```python
from build123d import *

# Parameters (mm, degrees)
SKETCH1_W           = 90
SKETCH1_H           = 60
BOSS_EXTRUDE1_DEPTH = 20
CUT_EXTRUDE1_DEPTH  = 61
SKETCH3_R           = 4.3
CUT_EXTRUDE2_DEPTH  = 21
SKETCH4_R           = 8.8
CUT_EXTRUDE3_DEPTH  = 10
CHAMFER1_SIZE       = 1


with BuildPart() as part:
    # Sketch1 → Boss-Extrude1 (new body)
    with BuildSketch(Plane(origin=(0, 0, 0), x_dir=(1, 0, 0), z_dir=(0, 1, 0))):
        Rectangle(SKETCH1_W, SKETCH1_H)
    extrude(amount=BOSS_EXTRUDE1_DEPTH)

    # Sketch2 → Cut-Extrude1 (cut, through all)
    with BuildSketch(Plane.XY.offset(30)):
        Polygon((28, 25), (-28, 25), (-28, 15), (-7.8, 15), (-7.8, 20), (7.8, 20), (7.8, 15), (28, 15), align=None)
    extrude(amount=-CUT_EXTRUDE1_DEPTH, mode=Mode.SUBTRACT)

    # Sketch3 → Cut-Extrude2 (cut, through all)
    with BuildSketch(Plane.XZ):
        with Locations((-35, 15)):
            Circle(SKETCH3_R)
        with Locations((-35, -15)):
            Circle(SKETCH3_R)
        with Locations((35, -14.217273236)):
            Circle(SKETCH3_R)
        with Locations((35, 15)):
            Circle(SKETCH3_R)
    extrude(amount=-CUT_EXTRUDE2_DEPTH, mode=Mode.SUBTRACT)

    # Sketch4 → Cut-Extrude3 (cut)
    with BuildSketch(Plane.XZ):
        with Locations((35, 15)):
            Circle(SKETCH4_R)
        with Locations((35, -14.217273236)):
            Circle(SKETCH4_R)
        with Locations((-35, 15)):
            Circle(SKETCH4_R)
        with Locations((-35, -15)):
            Circle(SKETCH4_R)
    extrude(amount=-CUT_EXTRUDE3_DEPTH, mode=Mode.SUBTRACT)

    # Chamfer1
    chamfer1_edges = [part.edges().sort_by_distance(p)[0] for p in [
        (28, 20, 0),
        (-28, 20, 0),
        (7.8, 20, 0),
        (-7.8, 20, 0),
    ]]
    chamfer(chamfer1_edges, length=CHAMFER1_SIZE)


solid = part.part
```
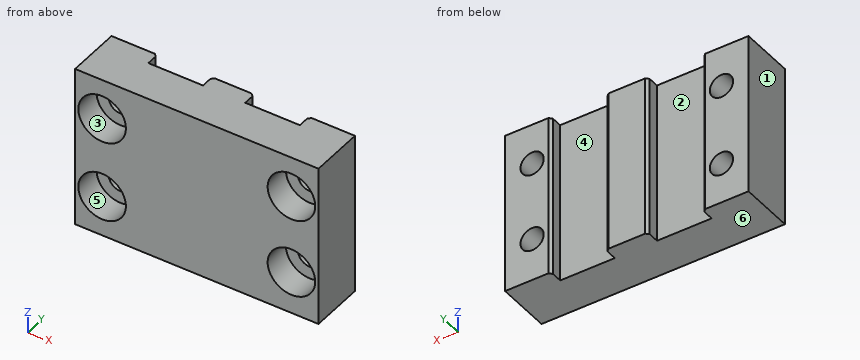
Check sheet for the modelled part. Datum: model origin and axes. Units: mm. Face numbers are marked on the shaded views. A direction names the side the tool comes from. Give positions to 0.01 mm unless a question says otherwise; leave off trailing zeros. Order: outer loops, then holes, each group sorted by start corner. A loop starts at its lowest first (then second) coordinate and runs counter-clockwise, first axis right, second up. Notation, with made-up numbers: (-10.5, 3) -> (17.5, 3) arc R16 ccw to (17.5, 33) -> close; hole circle Ø10 at (80, 80.5). An arc over 180 degrees is marked (long way). Return JSON: item names as keys, results as strings.
1. Cross-section at B-B, the plane z = 15. Count the separate pieces of the cut face and the enclosed holes in it, plus the area to 3 significant figures.
From the geometry:
{"separate pieces": "3", "enclosed holes": "0", "area": "1,070 mm^2"}
2. Material ranges on probe 1 along X at (y, z) = (17.5, 20); probe 2 along Z at (x, y) = (35, 16.75); probe 3 along Z at (x, y) = (-35, 3.25), recorded low to high. Write a range as [from, to].
From the geometry:
{"probe 1": "[-45, -28], [-7.8, 7.8], [28, 45]", "probe 2": "[-30, -18.52], [-9.92, 10.7], [19.3, 30]", "probe 3": "[-30, -23.8], [-6.2, 6.2], [23.8, 30]"}
3. Set-up check for the marked faces 1, 2 and 3: record each of +Z, -Z, +X, -X, +Y, -Y from which the full face is reachable in a straight line by a thin tool's end or side.
From the geometry:
{"face 1": "+Z, -Z, -X, +Y, -Y", "face 2": "+Z, -Z, +Y", "face 3": "-Y"}
4. Mould release check, pull along Z, two halves, no side actions. Record for the marked faces 4, 5 and 6: +Z half, -Z half, draft (parallel to the pull), parting line (faces both ways), or undercut.
From the geometry:
{"face 4": "draft", "face 5": "undercut", "face 6": "-Z half"}
5. Cross-section at C-C, the plane y = 3.75. Record the cut outline in (x, z), plus the area to 3 significant figures.
From the geometry:
{"outline": "(-45, -30) -> (45, -30) -> (45, 30) -> (-45, 30) -> close; hole circle Ø17.6 at (-35, -15); hole circle Ø17.6 at (-35, 15); hole circle Ø17.6 at (35, -14.22); hole circle Ø17.6 at (35, 15)", "area": "4,430 mm^2"}
6. Go/stop test with flat-tipped pins: P1, Ø1.5, axis at x = -24, z = 4.5, coming from the -Y side; P2, Ø14, axis at x = -35.5, z = -16, coming from the -Y side; P3, Ø2, axis at x = 10.5, z = -6, coming from the +Y side. Record where each tip stops, or that it passes through.
From the geometry:
{"P1": "y = 0", "P2": "y = 10", "P3": "y = 15"}
7. Cross-section at D-D, the plane z = 3.5. Record the cut outline in (x, y).
From the geometry:
{"outline": "(-45, 0) -> (45, 0) -> (45, 20) -> (29, 20) -> (28, 19) -> (28, 15) -> (7.8, 15) -> (7.8, 19) -> (6.8, 20) -> (-6.8, 20) -> (-7.8, 19) -> (-7.8, 15) -> (-28, 15) -> (-28, 19) -> (-29, 20) -> (-45, 20) -> close"}
8. Cross-section at A-A, the plane x = 35. Record the cut outline in (y, z).
From the geometry:
{"outline": "(0, -30) -> (20, -30) -> (20, -18.52) -> (10, -18.52) -> (10, -23.02) -> (0, -23.02) -> close; (0, -5.42) -> (10, -5.42) -> (10, -9.92) -> (20, -9.92) -> (20, 10.7) -> (10, 10.7) -> (10, 6.2) -> (0, 6.2) -> close; (0, 23.8) -> (10, 23.8) -> (10, 19.3) -> (20, 19.3) -> (20, 30) -> (0, 30) -> close"}
